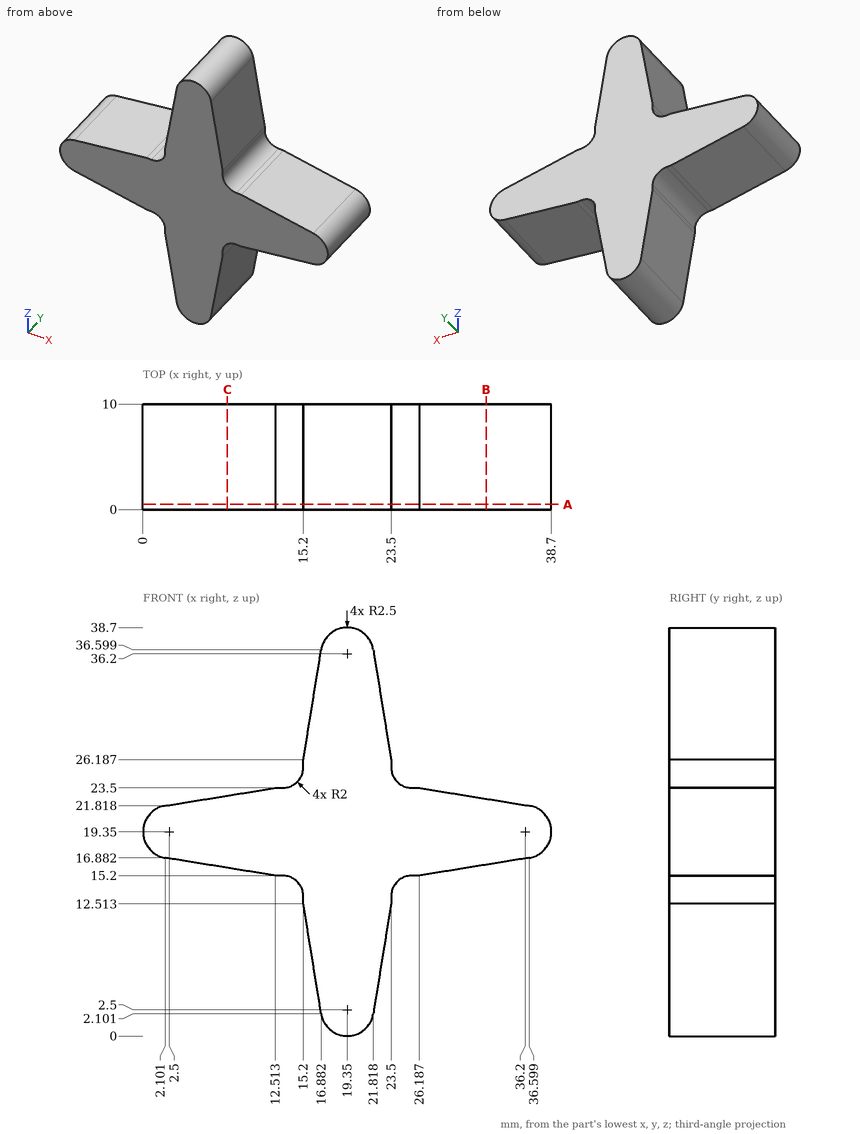
Geometry: see drawing. Coordinates: mm, zero at the bounding-box minimum. Give positions to 0.01 mm unless a question says otherwise; leave off trailing zeros. Loops run counter-clockwise (first coordinate to the right, second up) from the corner with the lowest first, then second, coordinate; pieces in that order, holes last. Notation, with made-up numbers: (73.25, 66.5) - (93.25, 66.5) arc R30 cw to (93.25, 90.5) - close; hole circle Ø2 at (-29.5, 0.5). An arc over 180 degrees is marked (long way). Answer as CSV lines item,"result". Start each with the question number.
1. Section B-B, the plane x = 32.5. Return loops of the section in (y, z), plus the area to 3 significant figures.
2. Ray query, L1, parallel to Z at x = 31, y = 7.25; L2, parallel to X at y = 4.5, z = 26; L3, parallel to Z at x = 21, y = 7.75. Return the intervals inside material, ascending.
3. Section A-A, the plane y = 0.5. Return loops of the section in (x, z).
4. Section C-C, the plane x = 8. Return loops of the section in (y, z), plus the area to 3 significant figures.
5. Pin query (flat end, axial travel): P1, Ø2, axis at y = 8, z = 26.5, coming from the +X side; P2, Ø0.8, axis at x = 13, y = 6, coming from the -Z side; P3, Ø3, axis at x = 5, y = 9, coming from the +Z side. Return the tip coordinate at first contact, or that it passes through.
Answers:
1,outline,"(0, 16.22) - (10, 16.22) - (10, 22.48) - (0, 22.48) - close"
1,area,"62.6 mm2"
2,L1,"z = 15.98 to 22.72"
2,L2,"x = 15.2 to 23.5"
2,L3,"z = 0.62 to 38.08"
3,outline,"(2.1, 16.88) - (12.51, 15.2) - (13.2, 15.2) arc R2 cw to (15.2, 13.2) - (15.2, 12.51) - (16.88, 2.1) arc R2.5 ccw to (21.82, 2.1) - (23.5, 12.51) - (23.5, 13.2) arc R2 cw to (25.5, 15.2) - (26.19, 15.2) - (36.6, 16.88) arc R2.5 ccw to (36.6, 21.82) - (26.19, 23.5) - (25.5, 23.5) arc R2 cw to (23.5, 25.5) - (23.5, 26.19) - (21.82, 36.6) arc R2.5 ccw to (16.88, 36.6) - (15.2, 26.19) - (15.2, 25.5) arc R2 cw to (13.2, 23.5) - (12.51, 23.5) - (2.1, 21.82) arc R2.5 ccw to start"
4,outline,"(0, 15.93) - (10, 15.93) - (10, 22.77) - (0, 22.77) - close"
4,area,"68.4 mm2"
5,P1,"stops at x = 23.5"
5,P2,"stops at z = 15.19"
5,P3,"stops at z = 22.53"
